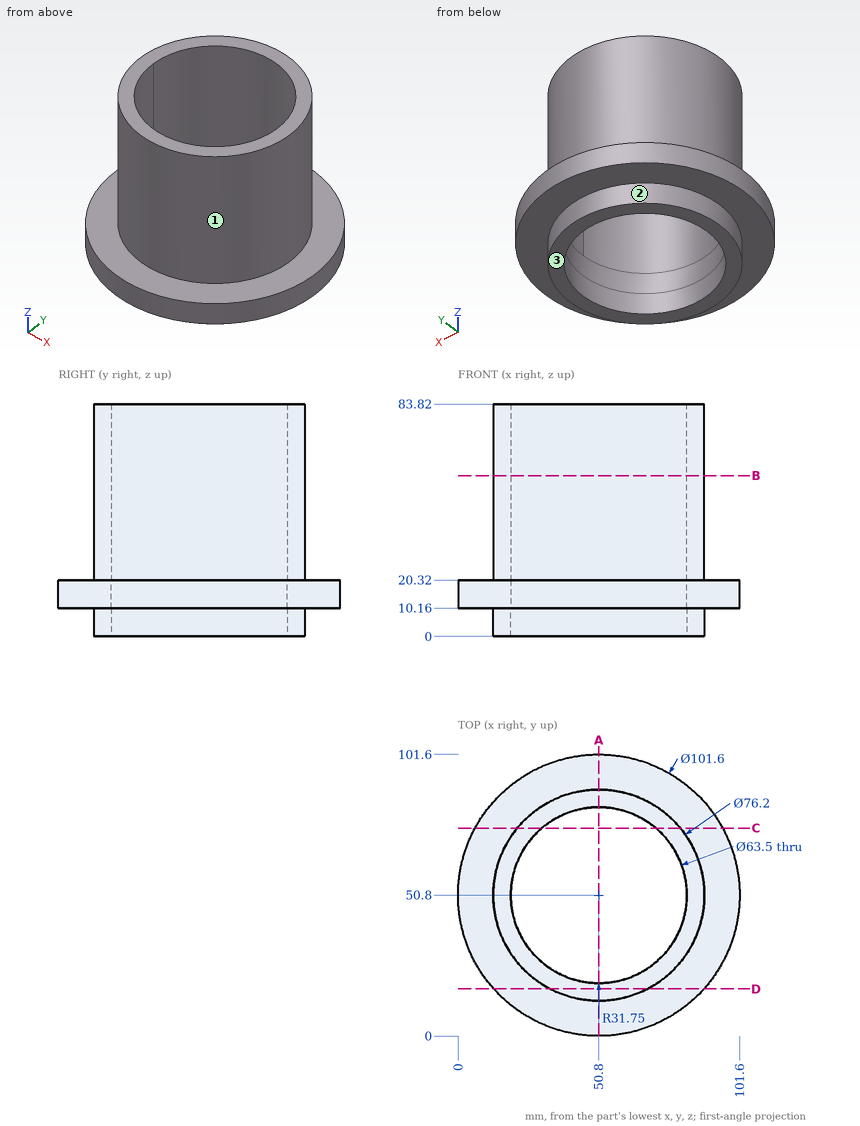
The figure shows three views and two pictorial views of one solid part (mm, origin at its lowest corner). Answer the questions. A direction names the side the tool comes from. Round coordinates to 2 decimals unless told otherwise and drop trailing zeros. Write each loop counter-clockwise with the first axis right and the second up, starting at its lowest first coordinate (ties: lowest second). Pieces come first, ordered by that corner, then holes. Notation, with made-up numbers: (69, 83) - (103, 83) arc R17 ccw to (103, 108) - close; hole circle Ø2 at (42, 60.25). An arc over 180 degrees is marked (long way). Answer in a Markdown table with one row per item. Add a question column.
1. A cutting plane is placed at D-D, the plane y = 17. Determine the outline of the cut face in (x, z), and give its area (3 significant figures).
2. A cutting plane is placed at B-B, the plane z = 58. Determine the outline of the cut face in (x, y).
3. A cutting plane is placed at C-C, the plane y = 75. Determine the outline of the cut face in (x, z), and give its area (3 significant figures).
4. A cutting plane is placed at A-A, the plane x = 50.8. Determine the outline of the cut face in (y, z), and give its area (3 significant figures).
5. For the marked faces 1, 2 and 3, determine the directions among +Z, -Z, +X, -X, +Y, -Y from which every point of the face is accessible in a straight line to the end or side of a thin tool.
6. Find the intervals of material crossed by line 1 along Y through (x, z) = (50, 16); line 2 along Y through (x, z) = (50.8, 7.75); line 3 along X through (y, z) = (28, 79), in increasing order. Write a range as from..to.
7. Given pin 1 (2 mm diameter, centred on x = 60, z = 75.5, fed in from +Y); pin 2 (8 mm diameter, centred on x = 91, y = 80, fed in from -Z); pin 3 (3 mm diameter, centred on y = 49.5, z = 74.5, fed in from -X); pin 4 (1.5 mm diameter, centred on y = 90.5, z = 55, fed in from -X), each flat-ended and moving along its own axis, determine where each tip first touches the part or whether it passes through.
Worked out:
| question | item | result |
|---|---|---|
| 1 | outline | (12.88, 10.16) - (33.22, 10.16) - (33.22, 0) - (68.38, 0) - (68.38, 10.16) - (88.72, 10.16) - (88.72, 20.32) - (68.38, 20.32) - (68.38, 83.82) - (33.22, 83.82) - (33.22, 20.32) - (12.88, 20.32) - close |
| 1 | area | 3,360 mm^2 |
| 2 | outline | circle Ø76.2 at (50.8, 50.8); hole circle Ø63.5 at (50.8, 50.8) |
| 3 | outline | (6.13, 10.16) - (21.37, 10.16) - (21.37, 0) - (30.25, 0) - (30.25, 83.82) - (21.37, 83.82) - (21.37, 20.32) - (6.13, 20.32) - close; (71.35, 0) - (80.23, 0) - (80.23, 10.16) - (95.47, 10.16) - (95.47, 20.32) - (80.23, 20.32) - (80.23, 83.82) - (71.35, 83.82) - close |
| 3 | area | 1,800 mm^2 |
| 4 | outline | (0, 10.16) - (12.7, 10.16) - (12.7, 0) - (19.05, 0) - (19.05, 83.82) - (12.7, 83.82) - (12.7, 20.32) - (0, 20.32) - close; (82.55, 0) - (88.9, 0) - (88.9, 10.16) - (101.6, 10.16) - (101.6, 20.32) - (88.9, 20.32) - (88.9, 83.82) - (82.55, 83.82) - close |
| 4 | area | 1,320 mm^2 |
| 5 | face 1 | +Z |
| 5 | face 2 | -Z |
| 5 | face 3 | -Z, +X, -X, +Y, -Y |
| 6 | line 1 | 0.01..19.06, 82.54..101.59 |
| 6 | line 2 | 12.7..19.05, 82.55..88.9 |
| 6 | line 3 | 20.28..28.7, 72.9..81.32 |
| 7 | pin 1 | y = 88.01 |
| 7 | pin 2 | z = 10.16 |
| 7 | pin 3 | x = 12.7 |
| 7 | pin 4 | through |
